Design review of the part built by this model. Coordinates are the model's own, in mm. Face numbers are marked on the shaded views. Coordinates: 2 decimals unless noted, no trailing zeros. Loops run counter-clockwise (first coordinate to the right, second up) from the corner with the lowest first, then second, coordinate; pieces in that order, holes last. Notation, with made-up numbers: (78.25, 18.25) - (133.25, 18.25) arc R21 cw to (133.25, 32.25) - close; hole circle Ø10 at (4.25, 55.5). An arc over 180 degrees is marked (long way). Answer in a Markdown table with one row per item. Add a question column.
(1) We need section A-A, the plane y = -12. Write out the cut boundary in (x, z), plus the area to 3 significant figures.
(2) To check wall thickness, follow L1, parallel to X at y = -11, z = 0.35; L2, parallel to Y at x = 28, z = 0.4; L3, parallel to Z at x = 14.5, y = 25.5. State the ranges of each line that lie inside material, in increasing order. Write a range as [from, to].
(3) The part is to be moulded in two halves that separate along X. For the marked faces 1 and 2, say which applies: released by +X, released by -X, zero draft, split by the parting line, or undercut.
(4) We need section C-C, the plane y = -31.5. Write out the cut boundary in (x, z).
(5) We need section D-D, the plane x = -38. Write out the cut boundary in (y, z).
(6) We need section B-B, the plane x = 41.5. Write out the cut boundary in (y, z), plus the area to 3 significant figures.
(7) Clearance check with flat-ended pins moving along their axes: pin 1 (4 mm diameter, centred on x = 27.5, y = 10, fed in from +Z); pin 2 (4 mm diameter, centred on x = -24.5, y = 26.5, fed in from +Z). State where each tip first meets the part, or that it passes through.
from build123d import *

# Parameters (mm, degrees)
F0_W     = 127
F0_H     = 88.9
F1_DEPTH = 0.3
F2_R     = 8
F2_R_2   = 3
F3_DEPTH = 0.3
F2_W     = 33.9999994338
F2_H     = 41.9999994338
F4_DEPTH = 0.6


with BuildPart() as f1:
    # F0 (on Top) → F1 (new body)
    with BuildSketch(Plane.XY):
        Rectangle(F0_W, F0_H)
    extrude(amount=F1_DEPTH)

    # F2 (on face) → F3 (join)
    with BuildSketch(Plane.XY.offset(0.3)):
        with Locations((-31.75, 0)):
            Circle(F2_R)
        with Locations((-29.3087995864, -1.7437145812)):
            Circle(F2_R_2, mode=Mode.SUBTRACT)
        with Locations((30.75, 0)):
            Circle(F2_R)
        with Locations((32.1912004136, -1.7437145812)):
            Circle(F2_R_2, mode=Mode.SUBTRACT)
        with BuildLine():
            Line((-42.75, 15), (-42.75, 7))
            ThreePointArc((-42.75, 7), (-37.0931457505, 9.3431457505), (-34.75, 15))
            Line((-34.75, 15), (-42.75, 15))
        make_face()
        with BuildLine():
            ThreePointArc((20.75, 7.0627460668), (27.0415026221, 9), (29.75, 15))
            Line((29.75, 15), (20.75, 15))
            Line((20.75, 15), (20.75, 7.0627460668))
        make_face()
        with Locations((-29.3087995864, -1.7437145812)):
            Circle(F2_R_2)
        with Locations((32.1912004136, -1.7437145812)):
            Circle(F2_R_2)
    extrude(amount=F3_DEPTH)

    # F2 (on face) → F4 (join)
    with BuildSketch(Plane.XY.offset(0.3)):
        with Locations((-31.75, 0)):
            Rectangle(F2_W, F2_H)
        Polygon((-20.75, 15), (-20.75, -15), (-42.75, -15), (-42.75, 7), (-42.75, 15), (-34.75, 15), align=None, mode=Mode.SUBTRACT)
        with Locations((31.75, 0)):
            Rectangle(F2_W, F2_H)
        Polygon((29.75, 15), (42.75, 15), (42.75, -15), (20.75, -15), (20.75, 7.0627460668), (20.75, 15), align=None, mode=Mode.SUBTRACT)
        with Locations((-29.3087995864, -1.7437145812)):
            Circle(F2_R_2)
        with Locations((32.1912004136, -1.7437145812)):
            Circle(F2_R_2)
    extrude(amount=F4_DEPTH)


solid = f1.part
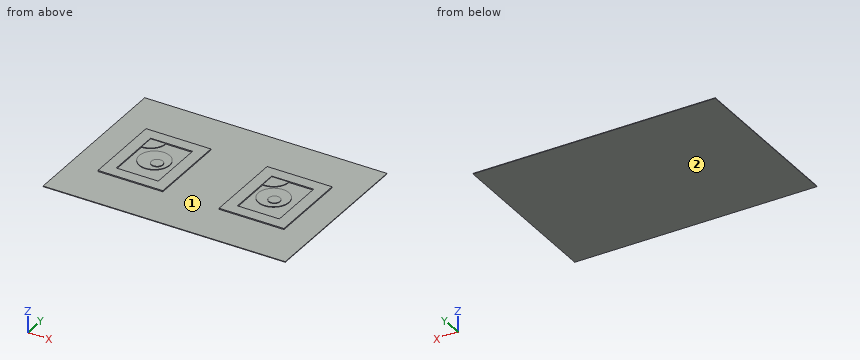
Responses:
| question | item | result |
|---|---|---|
| 1 | outline | (-63.5, 0) - (63.5, 0) - (63.5, 0.3) - (48.75, 0.3) - (48.75, 0.9) - (42.75, 0.9) - (42.75, 0.3) - (20.75, 0.3) - (20.75, 0.9) - (14.75, 0.9) - (14.75, 0.3) - (-14.75, 0.3) - (-14.75, 0.9) - (-20.75, 0.9) - (-20.75, 0.3) - (-42.75, 0.3) - (-42.75, 0.9) - (-48.75, 0.9) - (-48.75, 0.3) - (-63.5, 0.3) - close |
| 1 | area | 52.5 mm2 |
| 2 | L1 | x = [-48.75, -42.75], [-20.75, -14.75], [14.75, 20.75], [42.75, 48.75] |
| 2 | L2 | y = [-21, -15], [-7.51, 7.51], [10.01, 21] |
| 2 | L3 | z = [0, 0.3] |
| 3 | face 1 | undercut |
| 3 | face 2 | zero draft |
| 4 | outline | (-63.5, 0) - (63.5, 0) - (63.5, 0.3) - (-63.5, 0.3) - close |
| 5 | outline | (-44.45, 0) - (44.45, 0) - (44.45, 0.3) - (21, 0.3) - (21, 0.9) - (15, 0.9) - (15, 0.6) - (8.56, 0.6) - (8.56, 0.3) - (4.99, 0.3) - (4.99, 0.6) - (-4.99, 0.6) - (-4.99, 0.3) - (-15, 0.3) - (-15, 0.9) - (-21, 0.9) - (-21, 0.3) - (-44.45, 0.3) - close |
| 6 | outline | (-44.45, 0) - (44.45, 0) - (44.45, 0.3) - (21, 0.3) - (21, 0.9) - (15, 0.9) - (15, 0.3) - (-15, 0.3) - (-15, 0.9) - (-21, 0.9) - (-21, 0.3) - (-44.45, 0.3) - close |
| 6 | area | 33.9 mm2 |
| 7 | pin 1 | stops at z = 0.6 |
| 7 | pin 2 | stops at z = 0.3 |
